Geometry: final body of the model. Coordinates: model frame, mm. A direction names the side the tool comes from. Coordinates: 2 decimals unless noted, no trailing zeros. Order: outer loops, then holes, each group sorted by start corner. A loop starts at its lowest first (then second) coordinate and runs counter-clockwise, first axis right, second up. Notation, with made-up numbers: (39, 58) - (83, 58) arc R22 ccw to (83, 65) - close; hole circle Ø2 at (50, -11.75). An arc over 180 degrees is marked (long way). Use a Markdown table: item, result. Add a question column.
Autodesk Inventor part; units mm, degrees
ref_plane "YZ Plane" through (0, 0, 0) normal (1, 0, 0) x (0, 1, 0)
ref_plane "XZ Plane" through (0, 0, 0) normal (0, 1, 0) x (-1, 0, 0)
ref_plane "XY Plane" through (0, 0, 0) normal (0, 0, 1) x (1, 0, 0)
sketch "Sketch1" plane through (0, 0, 0) normal (0, 0, 1) x (1, 0, 0)
  line L0 (49, 21) -> (-49, 21)
  line L1 (-49, -21) -> (-21, -21)
  circle A0 centre (32, 0) radius 3.9
  circle A1 centre (-32, 0) radius 3.9
  line L2 (49, 21) -> (49, 10.5)
  line L3 (-49, -21) -> (-49, -10.5)
  line L4 (0, 41.7106) -> (0, -39.2634) construction
  line L5 (-50.5476, 0) -> (60.8869, 0) construction
  circle A2 centre (0, 0) radius 11.5
  line L6 (21, 21) -> (21, -21) construction
  line L7 (-21, -21) -> (-21, 21) construction
  line L8 (49, 21) -> (52, 21)
  line L9 (52, 21) -> (52, 10.5)
  line L10 (52, -21) -> (49, -21)
  line L11 (49, 10.5) -> (52, 10.5)
  line L12 (49, -10.5) -> (52, -10.5)
  line L13 (49, 10.5) -> (49, -10.5)
  line L14 (49, -10.5) -> (49, -21)
  line L15 (52, -10.5) -> (52, -21)
  line L16 (52, 10.5) -> (52, -10.5)
  line L17 (44.6, 2.65) -> (47, 2.65)
  line L18 (47, 2.65) -> (47, -2.65)
  line L19 (47, -2.65) -> (44.6, -2.65)
  line L20 (44.6, -2.65) -> (44.6, 2.65)
  line L21 (-49, 21) -> (-52, 21)
  line L22 (-52, 21) -> (-52, 10.5)
  line L23 (-49, 10.5) -> (-52, 10.5)
  line L24 (-49, -10.5) -> (-52, -10.5)
  line L25 (-52, -10.5) -> (-52, -21)
  line L26 (-52, 10.5) -> (-52, -10.5)
  line L27 (-44.6, 2.65) -> (-47, 2.65)
  line L28 (-47, 2.65) -> (-47, -2.65)
  line L29 (-47, -2.65) -> (-44.6, -2.65)
  line L30 (-44.6, -2.65) -> (-44.6, 2.65)
  line L31 (-52, -21) -> (-49, -21)
  line L32 (-49, 10.5) -> (-49, 21)
  line L33 (-49, -10.5) -> (-49, 10.5)
  line L34 (52, -21) -> (52, -24)
  line L35 (52, -24) -> (-52, -24)
  line L36 (-52, -24) -> (-52, -21)
  line L37 (34.6667, -24) -> (34.6667, -21)
  line L38 (-34.6667, -24) -> (-34.6667, -21)
  line L39 (-2.65, -16.6) -> (2.65, -16.6)
  line L40 (2.65, -16.6) -> (2.65, -19)
  line L41 (2.65, -19) -> (-2.65, -19)
  line L42 (-2.65, -19) -> (-2.65, -16.6)
  line L43 (21, -21) -> (49, -21)
  line L44 (-21, -21) -> (21, -21)
  circle A3 centre (-15.5, 15.5) radius 1.4
  circle A4 centre (-15.5, -15.5) radius 1.4
  circle A5 centre (15.5, -15.5) radius 1.4
  circle A6 centre (15.5, 15.5) radius 1.4
  dimension "d4" = 7.8
  dimension "d5" = 7.8
  dimension "d111" = 42
  dimension "d115" = 21
  dimension "d116" = 21
  dimension "d117" = 23
  dimension "d118" = 42
  dimension "d123" = 3
  dimension "d124" = 21
  dimension "d125" = 5.3
  dimension "d126" = 2.4
  dimension "d128" = 5
  dimension "d129" = 3
  dimension "d130" = 104
  dimension "d131" = 69.3333
  dimension "d132" = 5.3
  dimension "d133" = 2.4
  dimension "d134" = 5
  dimension "d135" = 2.8
  dimension "d136" = 5.5
  dimension "d137" = 5.5
  dimension "d140" = 360
  dimension "d143" = 12.6
extrude "Extrusion1" add sketch "Sketch1" against normal blind 3 contours L2 L13 L14 L43 L44 L1 L3 L33 L32 L0 | L8 L9 L11 L2 | L32 L23 L22 L21 | L12 L15 L10 L14 | L3 L31 L25 L24 | L10 L34 L35 L37 L43 | L1 L38 L35 L36 L31
properties part number "X-Motor-Housing_Front-Inner"
1) Access query for faces 1 (the flat face through (-50, 10.5, -1)), 2 (the flat face through (50, -10.5, -1)), 3 (the flat face through (-52, 16, -1)), 4 (the flat face through (34.667, -23, -1)), 5 (the flat face through (0, -16.6, -1)). Directions: +Z, -Z, +X, -X, +Y, -Y. A direction counts if a zero-diameter tool reaches every point of the face in a straight line with its end or side. Return the directions, or none.
2) Section query D-D (y = -7.5). Return the cut outline in (x, z), and give its area (3 significant figures).
3) Section query A-A (x = -15.5). Return the cut outline in (y, z), and give its area (3 significant figures).
4) Section query C-C (x = 32). Return the cut outline in (y, z), and give its area (3 significant figures).
5) Draft query along Y for faces 6 (the flat face through (46, 2.65, -1)), 7 (the flat face through (-52, -17, -1)), 8 (the flat face through (-47, 0, -1)), 9 (the flat face through (43, -24, -1)). Return one class per face: released by +Y, released by -Y, zero draft, split by the parting line, or undercut.
6) Line query: line 1 (Y direction, x = -15.5, z = -1.65); line 2 (Y direction, x = -0.5, z = -0.55); line 3 (X direction, y = -17, z = -0.25). Output: solid intervals per line, ascending. Write a range as from..to.
7) First-contact query: pin 1 (1.5 mm diameter, centred on y = 4.5, z = -1, fed in from +X); pin 2 (0.9 mm diameter, centred on y = 0, z = -1.5, fed in from -X); pin 3 (12 mm diameter, centred on x = 12, y = -8, fed in from +Z). Flat tips, straight axial feed; report the tip coordinate or a pass-through.
8) Section query B-B (y = -15.5). Return the cut outline in (x, z).
From the geometry:
| question | item | result |
|---|---|---|
| 1 | face 1 | +Z, -Z, -X |
| 1 | face 2 | +Z, -Z, +X |
| 1 | face 3 | +Z, -Z, -X, +Y, -Y |
| 1 | face 4 | +Z, -Z, -Y |
| 1 | face 5 | +Z, -Z |
| 2 | outline | (-49, -3) - (-8.72, -3) - (-8.72, 0) - (-49, 0) - close; (8.72, -3) - (49, -3) - (49, 0) - (8.72, 0) - close |
| 2 | area | 242 mm^2 |
| 3 | outline | (-21, -3) - (-16.9, -3) - (-16.9, 0) - (-21, 0) - close; (-14.1, -3) - (14.1, -3) - (14.1, 0) - (-14.1, 0) - close; (16.9, -3) - (21, -3) - (21, 0) - (16.9, 0) - close |
| 3 | area | 109 mm^2 |
| 4 | outline | (-21, -3) - (-3.9, -3) - (-3.9, 0) - (-21, 0) - close; (3.9, -3) - (21, -3) - (21, 0) - (3.9, 0) - close |
| 4 | area | 103 mm^2 |
| 5 | face 6 | undercut |
| 5 | face 7 | zero draft |
| 5 | face 8 | undercut |
| 5 | face 9 | released by -Y |
| 6 | line 1 | y = -21..-16.9, -14.1..14.1, 16.9..21 |
| 6 | line 2 | y = -21..-19, -16.6..-11.49, 11.49..21 |
| 6 | line 3 | x = -52..-2.65, 2.65..52 |
| 7 | pin 1 | stops at x = 49 |
| 7 | pin 2 | stops at x = -49 |
| 7 | pin 3 | stops at z = 0 |
| 8 | outline | (-52, -3) - (-16.9, -3) - (-16.9, 0) - (-52, 0) - close; (-14.1, -3) - (14.1, -3) - (14.1, 0) - (-14.1, 0) - close; (16.9, -3) - (52, -3) - (52, 0) - (16.9, 0) - close |
